```python
from build123d import *

# Parameters (mm, degrees)
CROQUIS1_W                   = 152
CROQUIS1_H                   = 85
SALIENTE_EXTRUIR1_DEPTH      = 1.5
CROQUIS2_W                   = 156
CROQUIS2_H                   = 89
CROQUIS2_W_2                 = 152
CROQUIS2_H_2                 = 85
SALIENTE_EXTRUIR3_DEPTH      = 5
SALIENTE_EXTRUIR3_DEPTH_BACK = 1.5
CROQUIS3_R                   = 2.75
SALIENTE_EXTRUIR4_DEPTH      = 3.5
CROQUIS4_W                   = 119.5
CROQUIS4_H                   = 78.5
CORTAR_EXTRUIR1_DEPTH        = 1.5
CROQUIS5_R                   = 1.5
CORTAR_EXTRUIR2_DEPTH        = 3


with BuildPart() as part:
    # Croquis1 → Saliente-Extruir1 (new body)
    with BuildSketch(Plane(origin=(0, 0, 0), x_dir=(1, 0, 0), z_dir=(0, 1, 0))):
        with Locations((76, 42.5)):
            Rectangle(CROQUIS1_W, CROQUIS1_H)
    extrude(amount=SALIENTE_EXTRUIR1_DEPTH)

    # Croquis2 → Saliente-Extruir3 (add, two sides)
    with BuildSketch(Plane(origin=(0, 1.5, 0), x_dir=(1, 0, 0), z_dir=(0, 1, 0))) as saliente_extruir3_sk:
        with Locations((76, 42.5)):
            Rectangle(CROQUIS2_W, CROQUIS2_H)
        with Locations((76, 42.5)):
            Rectangle(CROQUIS2_W_2, CROQUIS2_H_2, mode=Mode.SUBTRACT)
    extrude(amount=SALIENTE_EXTRUIR3_DEPTH)
    extrude(saliente_extruir3_sk.sketch, amount=-SALIENTE_EXTRUIR3_DEPTH_BACK)

    # Croquis3 → Saliente-Extruir4 (add)
    with BuildSketch(Plane(origin=(0, 1.5, 0), x_dir=(1, 0, 0), z_dir=(0, 1, 0))):
        with Locations((3, 82)):
            Circle(CROQUIS3_R)
        with Locations((3, 3)):
            Circle(CROQUIS3_R)
        with Locations((130, 82)):
            Circle(CROQUIS3_R)
        with Locations((130, 3)):
            Circle(CROQUIS3_R)
    extrude(amount=SALIENTE_EXTRUIR4_DEPTH)

    # Croquis4 → Cortar-Extruir1 (cut)
    with BuildSketch(Plane.XZ):
        with Locations((67.35, -41.25)):
            Rectangle(CROQUIS4_W, CROQUIS4_H)
    extrude(amount=-CORTAR_EXTRUIR1_DEPTH, mode=Mode.SUBTRACT)

    # Croquis5 → Cortar-Extruir2 (cut)
    with BuildSketch(Plane(origin=(0, 5, 0), x_dir=(1, 0, 0), z_dir=(0, 1, 0))):
        with Locations((130, 3)):
            Circle(CROQUIS5_R)
        with Locations((3, 3)):
            Circle(CROQUIS5_R)
        with Locations((3, 82)):
            Circle(CROQUIS5_R)
        with Locations((130, 82)):
            Circle(CROQUIS5_R)
    extrude(amount=-CORTAR_EXTRUIR2_DEPTH, mode=Mode.SUBTRACT)


solid = part.part
```
For this review, take the finished solid that the model builds, in its own axes (mm). Coordinates: 2 decimals unless noted, no trailing zeros. Write each loop counter-clockwise with the first axis right and the second up, starting at its lowest first coordinate (ties: lowest second). Pieces come first, ordered by that corner, then holes. Notation, with made-up numbers: (19.5, -4.75) - (76.5, -4.75) arc R15 ccw to (76.5, 11.25) - close; hole circle Ø2 at (-5.5, 15.5). An arc over 180 degrees is marked (long way). Put each result on its own line as item: value.
1. Add section A-A, the plane y = 3.25. Count the separate pieces of the cut face and the enclosed holes in it, then the cut area to 3 significant figures.
Values found:
separate pieces: 5
enclosed holes: 5
area: 1,030 mm²
2. For pin 1 (1.5 mm diameter, centred on x = 2.5, z = -82.5, fed in from +Y); pin 2 (3.5 mm diameter, centred on x = 130.5, z = -3.5, fed in from +Y); pin 3 (10 mm diameter, centred on x = 136.5, z = -68.5, fed in from +Y), all flat-tipped, find the tip position at first contact; note any pin that passes through.
Values found:
pin 1: y = 2
pin 2: y = 5
pin 3: y = 1.5
3. Add section B-B, the plane x = 74. Give the boundary of the cut face in (y, z), then the cut area to 4 significant figures.
Values found:
outline: (0, -87) - (6.5, -87) - (6.5, -85) - (1.5, -85) - (1.5, -80.5) - (0, -80.5) - close; (0, -2) - (1.5, -2) - (1.5, 0) - (6.5, 0) - (6.5, 2) - (0, 2) - close
area: 35.75 mm²
4. Mouldability with a two-part tool opening along X and no side actions: class faces 1 (the flat face through (-2, 3, -42)), 2 (the flat face through (75, 4, 0)), 3 (the flat face through (154, 3, -42)) as released by +X, released by -X, zero draft, split by the parting line, or undercut.
Values found:
face 1: released by -X
face 2: undercut
face 3: released by +X
5. Wall thickness on probe 1 along X at (y, z) = (3.05, -3); probe 2 along X at (y, z) = (6, -11); probe 3 along Z at (x, y) = (3, 3): over which ranges is each line inside the solid? List them lowest first.
Values found:
probe 1: -2 to 0, 0.25 to 1.5, 4.5 to 5.75, 127.25 to 128.5, 131.5 to 132.75, 152 to 154
probe 2: -2 to 0, 152 to 154
probe 3: -87 to -85, -84.75 to -83.5, -80.5 to -79.25, -5.75 to -4.5, -1.5 to -0.25, 0 to 2
6. Add section D-D, the plane z = -82. Give the boundary of the cut face in (x, y), then the cut area to 4 significant figures.
Values found:
outline: (-2, 0) - (154, 0) - (154, 6.5) - (152, 6.5) - (152, 1.5) - (132.75, 1.5) - (132.75, 5) - (131.5, 5) - (131.5, 2) - (128.5, 2) - (128.5, 5) - (127.25, 5) - (127.25, 1.5) - (5.75, 1.5) - (5.75, 5) - (4.5, 5) - (4.5, 2) - (1.5, 2) - (1.5, 5) - (0.25, 5) - (0.25, 1.5) - (0, 1.5) - (0, 6.5) - (-2, 6.5) - close
area: 274.5 mm²
7. Add section C-C, the plane z = -7.5. Give the boundary of the cut face in (x, y), then the cut area to 4 significant figures.
Values found:
outline: (-2, 0) - (7.6, 0) - (7.6, 1.5) - (0, 1.5) - (0, 6.5) - (-2, 6.5) - close; (127.1, 0) - (154, 0) - (154, 6.5) - (152, 6.5) - (152, 1.5) - (127.1, 1.5) - close
area: 74.75 mm²
